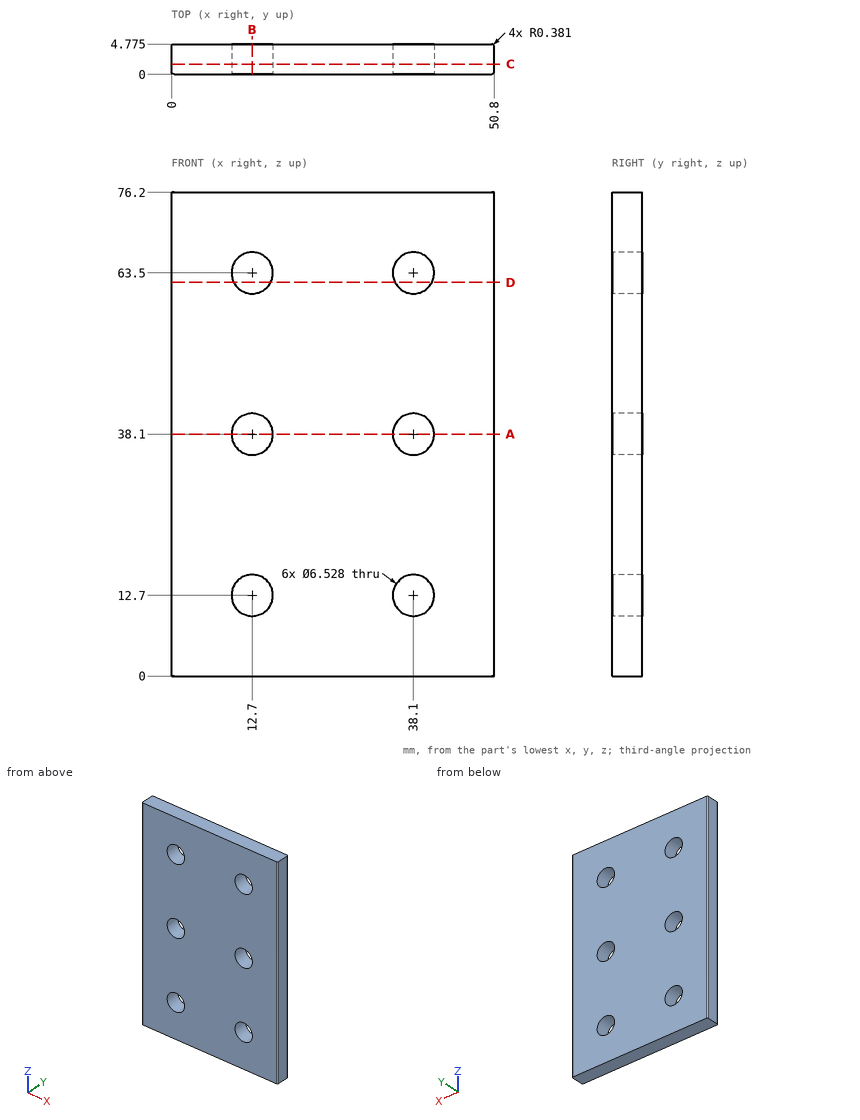
Geometry check sheet. Reference: drawing and pictorial views, mm from the part's lowest x, y, z. Give positions to 0.01 mm unless a question says otherwise; leave off trailing zeros. Write each loop counter-clockwise with the first axis right and the second up, starting at its lowest first coordinate (ties: lowest second). Pieces come first, ordered by that corner, then holes. Notation, with made-up numbers: M 18,87 L 23,87 A9 cw 23,100 Z; hole C 5,78.25 d7. An arc over 180 degrees is marked long. Answer as CSV lines item,"result". Start each with the question number.
Q1. Material ranges on L1, parallel to Z at x = 38.1, y = 2.9; L2, parallel to Z at x = 13, y = 4.15; L3, parallel to X at y = 0.95, z = 40.5, recorded low to high.
Q2. Section check B-B, the plane x = 12.7. Record the cut outline in (y, z) (1 decimal).
Q3. Section check A-A, the plane z = 38.1. Record the cut outline in (x, y) (1 decimal).
Q4. Section check C-C, the plane y = 1.6. Record the cut outline in (x, z), then the cut area to 3 significant figures.
Q5. Go/stop test with a flat-tipped pin: pin 1 (5 mm diameter, centred on x = 38.1, z = 63.5, fed in from +Y). Record where the tip stops, or that it passes through.
Q6. Section check D-D, the plane z = 62. Record the cut outline in (x, y) (1 decimal), then the cut area to 3 significant figures.
Geometry says:
1,L1,"0 to 9.44, 15.96 to 34.84, 41.36 to 60.24, 66.76 to 76.2"
1,L2,"0 to 9.45, 15.95 to 34.85, 41.35 to 60.25, 66.75 to 76.2"
1,L3,"0 to 10.49, 14.91 to 35.89, 40.31 to 50.8"
2,outline,"M 0,0 L 4.8,0 L 4.8,9.4 L 0,9.4 Z; M 0,16 L 4.8,16 L 4.8,34.8 L 0,34.8 Z; M 0,41.4 L 4.8,41.4 L 4.8,60.2 L 0,60.2 Z; M 0,66.8 L 4.8,66.8 L 4.8,76.2 L 0,76.2 Z"
3,outline,"M 0,0.4 A0.4 ccw 0.4,0 L 9.4,0 L 9.4,4.8 L 0.4,4.8 A0.4 ccw 0,4.4 Z; M 16,0 L 34.8,0 L 34.8,4.8 L 16,4.8 Z; M 41.4,0 L 50.4,0 A0.4 ccw 50.8,0.4 L 50.8,4.4 A0.4 ccw 50.4,4.8 L 41.4,4.8 Z"
4,outline,"M 0,0 L 50.8,0 L 50.8,76.2 L 0,76.2 Z; hole C 12.7,12.7 d6.53; hole C 12.7,38.1 d6.53; hole C 12.7,63.5 d6.53; hole C 38.1,12.7 d6.53; hole C 38.1,38.1 d6.53; hole C 38.1,63.5 d6.53"
4,area,"3,670 mm^2"
5,pin 1,"through"
6,outline,"M 0,0.4 A0.4 ccw 0.4,0 L 9.8,0 L 9.8,4.8 L 0.4,4.8 A0.4 ccw 0,4.4 Z; M 15.6,0 L 35.2,0 L 35.2,4.8 L 15.6,4.8 Z; M 41,0 L 50.4,0 A0.4 ccw 50.8,0.4 L 50.8,4.4 A0.4 ccw 50.4,4.8 L 41,4.8 Z"
6,area,"187 mm^2"
